Work out the finished part from the listing and answer in its coordinate system (mm). Face numbers are marked on the shaded views. A direction names the side the tool comes from. Coordinates: 2 decimals unless noted, no trailing zeros. Write each loop counter-clockwise with the first axis right and the second up, starting at its lowest first coordinate (ties: lowest second). Pieces come first, ordered by that corner, then holes. Notation, with made-up numbers: (-31.75, 79) - (-23.75, 79) arc R14 cw to (-23.75, 92) - close; hole circle Ø9 at (-38.5, 45.5). An arc over 180 degrees is marked (long way). Use a Markdown table: item, result. Add a question column.
(1) The part is cut by section A-A, the plane y = 14. Give the vertices of the cut face in (x, z), then the cut area to 3 significant figures.
(2) The part is cut by section D-D, the plane y = -5. Give the vertices of the cut face in (x, z).
(3) For a pull along Z with two mould halves and no side action, classify the marked faces 1, 2, 3 and 4 as released by +Z, released by -Z, zero draft, split by the parting line, or undercut.
(4) A tool of negligible diameter and unlimited length cuts with its end or side. For the marked faces 5, 6 and 7, from which of +Z, -Z, +X, -X, +Y, -Y can it reach the whole face along a straight path? Write none if from no direction.
(5) The part is cut by section B-B, the plane z = 5. Give the vertices of the cut face in (x, y).
(6) The part is cut by section C-C, the plane x = 0. Give the vertices of the cut face in (y, z), then the cut area to 3 significant figures.
(7) Find the intervals of material crossed by line 1 (X direction, y = 14, z = 0.5); line 2 (Y direction, x = 3.5, z = -7.25); line 3 (X direction, y = -3, z = -2.25), in increasing order. Write a range as from..to.
(8) Given pin 1 Ø1 at (x, z) = (-3, -2) entering from -Y; pin 2 Ø3 at (x, z) = (-1, 3.5) entering from -Y; pin 3 Ø0.8 at (x, z) = (0, -1) entering from +Y; pin 4 Ø1.6 at (x, z) = (0.5, 1) entering from +Y, each flat-ended and moving along its own axis, determine where each tip first touches the part or whether it passes through.
Autodesk Inventor part; units mm, degrees
ref_plane "YZ Plane" through (0, 0, 0) normal (1, 0, 0) x (0, 1, 0)
ref_plane "XZ Plane" through (0, 0, 0) normal (0, 1, 0) x (-1, 0, 0)
ref_plane "XY Plane" through (0, 0, 0) normal (0, 0, 1) x (1, 0, 0)
sketch "스케치1" plane through (0, 0, 0) normal (0, 1, 0) x (-1, 0, 0)
  arc A0 (5, 6) -> (-5, 6) centre (0, 6) ccw
  arc A1 (-5, -6) -> (5, -6) centre (0, -6) ccw
  line L0 (5, 6) -> (5, -6)
  line L1 (-5, 6) -> (-5, -6)
  point P0 (0, 0)
extrude "돌출1" add sketch "스케치1" along normal blind 20
sketch "스케치2" plane through (0, 20, 0) normal (0, 1, 0) x (1, 0, 0)
  line L0 (0, 0) -> (0, 3)
  line L1 (0, 3) -> (0, -3)
  circle A0 centre (0, 3) radius 1
  circle A1 centre (0, -3) radius 1
  line L2 (1, 3) -> (1, -3)
  line L3 (-1, -3) -> (-1, 3)
  dimension "d10" = 3
  dimension "d11" = 6
  dimension "d12" = 2
  dimension "d13" = 2
extrude "돌출2" cut sketch "스케치2" against normal blind 8
sketch "스케치3" plane through (0, 0, 0) normal (0, -1, 0) x (1, 0, 0)
  line L0 (-3, 0) -> (-3, 5.5316)
  line L1 (-2.6402, 6.2998) -> (-0.6402, 7.9665)
  line L2 (-3, 0) -> (-3, -5.5316)
  line L3 (-2.6402, -6.2998) -> (-0.6402, -7.9665)
  line L4 (3, 0) -> (3, 5.5316)
  line L5 (3, 5.5316) -> (3, -5.5316)
  line L6 (2.6402, -6.2998) -> (0.6402, -7.9665)
  line L7 (2.6402, 6.2998) -> (0.6402, 7.9665)
  arc A0 (-0.6402, -7.9665) -> (0.6402, -7.9665) centre (0, -7.1983) ccw
  arc A1 (2.6402, -6.2998) -> (3, -5.5316) centre (2, -5.5316) ccw
  arc A2 (3, 5.5316) -> (2.6402, 6.2998) centre (2, 5.5316) ccw
  arc A3 (0.6402, 7.9665) -> (-0.6402, 7.9665) centre (0, 7.1983) ccw
  arc A4 (-3, -5.5316) -> (-2.6402, -6.2998) centre (-2, -5.5316) ccw
  arc A5 (-2.6402, 6.2998) -> (-3, 5.5316) centre (-2, 5.5316) ccw
  point P0 (0, 0)
  point P1 (-3, -6)
  point P2 (3, -6)
  dimension "d24" = 1
extrude "돌출3" add sketch "스케치3" along normal blind 8
sketch "스케치4" plane through (0, -8, 0) normal (0, -1, 0) x (1, 0, 0)
  line L0 (0, 0) -> (0, 5)
  line L1 (0, 5) -> (0, -5)
  circle A0 centre (0, 5) radius 1
  circle A1 centre (0, -4.7812) radius 1
  dimension "d27" = 5
  dimension "d28" = 10
  dimension "d29" = 2
  dimension "d30" = 2
extrude "돌출4" add sketch "스케치4" along normal blind 8
ref_plane "작업 평면1" through (0, -16, 4) normal (-1, 0, 0) x (0, 0, 1)
sketch "스케치6" plane through (0, -16, 4) normal (-1, 0, 0) x (0, 0, 1)
  line L0 (0, 0) -> (2, 0)
  line L1 (0, -1) -> (1, -1)
  arc A0 (0, 0) -> (1, -1) centre (1, 0) ccw
  line L2 (1, -1) -> (1, 0)
  line L3 (1, 0) -> (0, 0)
  point P0 (-4, 16)
  point P1 (1, 0)
  point P2 (1, 0)
  dimension "d35" = 1
revolve "회전1" add sketch "스케치6" angle 360 about axis through (0, -17, 5) along (0, 1, 0)
sketch "스케치7" plane through (0, -16, 4) normal (-1, 0, 0) x (0, 0, 1)
  line L0 (-9.7812, 0) -> (-7.7812, 0)
  line L1 (-7.7812, 0) -> (-8.7812, 0)
  line L2 (-8.7812, 0) -> (-8.7812, -1)
  arc A0 (-8.7812, -1) -> (-7.7812, 0) centre (-8.7812, 0) ccw
  point P0 (-4, 16)
  dimension "d37" = 1
  dimension "d38" = 1
revolve "회전2" add sketch "스케치7" angle 360 about axis through (0, -16, -4.7812) along (0, -1, 0)
sketch "스케치8" plane through (0, 12, 0) normal (0, 1, 0) x (1, 0, 0)
  line L0 (0, 0) -> (0, 3)
  line L1 (0, 3) -> (0, -3)
  circle A0 centre (0, -3) radius 0.5
  circle A1 centre (0, 3) radius 0.5
  line L2 (-0.5, -3) -> (-0.5, 3)
  line L3 (0.5, -3) -> (0.5, 3)
  dimension "d40" = 3
  dimension "d41" = 6
  dimension "d42" = 1
  dimension "d43" = 1
extrude "돌출6" add sketch "스케치8" along normal blind 6
properties part number "Ctype addapter"
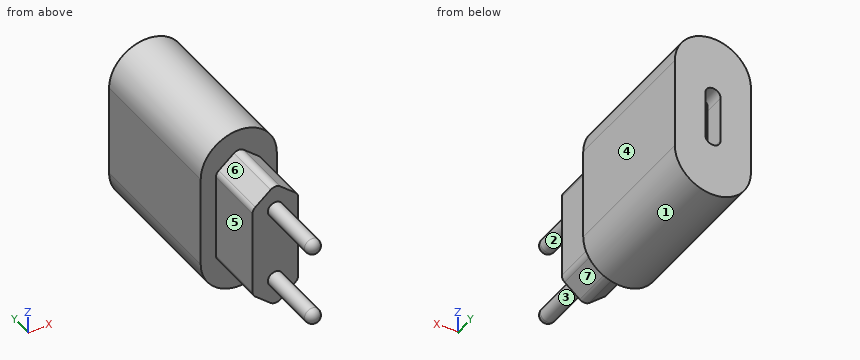
Model answer:
| question | item | result |
|---|---|---|
| 1 | outline | (-5, -6) arc R5 ccw to (5, -6) - (5, 6) arc R5 ccw to (-5, 6) - close; (-0.5, -3) arc R0.5 ccw to (0.5, -3) - (0.5, 3) arc R0.5 ccw to (-0.5, 3) - close; hole (-1, -3) arc R1 ccw to (1, -3) - (1, 3) arc R1 ccw to (-1, 3) - close |
| 1 | area | 190 mm^2 |
| 2 | outline | (-3, -5.53) arc R1 ccw to (-2.64, -6.3) - (-0.64, -7.97) arc R1 ccw to (0.64, -7.97) - (2.64, -6.3) arc R1 ccw to (3, -5.53) - (3, 5.53) arc R1 ccw to (2.64, 6.3) - (0.64, 7.97) arc R1 ccw to (-0.64, 7.97) - (-2.64, 6.3) arc R1 ccw to (-3, 5.53) - close |
| 3 | face 1 | released by -Z |
| 3 | face 2 | undercut |
| 3 | face 3 | undercut |
| 3 | face 4 | zero draft |
| 4 | face 5 | +Z, -Z, -X, -Y |
| 4 | face 6 | +Z, -X, -Y |
| 4 | face 7 | -Z, +X, -Y |
| 5 | outline | (-5, 0) - (-3, 0) - (-3, -8) - (-1, -8) - (-1, -16) arc R1 ccw to (1, -16) - (1, -8) - (3, -8) - (3, 0) - (5, 0) - (5, 20) - (-5, 20) - close |
| 6 | outline | (-16, -5.78) - (-8, -5.78) - (-8, -8.2) - (0, -8.2) - (0, -11) - (20, -11) - (20, -4) - (12, -4) - (12, -3.5) - (18, -3.5) - (18, 3.5) - (12, 3.5) - (12, 4) - (20, 4) - (20, 11) - (0, 11) - (0, 8.2) - (-8, 8.2) - (-8, 6) - (-16, 6) arc R1 ccw to (-16, 4) - (-8, 4) - (-8, -3.78) - (-16, -3.78) arc R1 ccw to start |
| 6 | area | 584 mm^2 |
| 7 | line 1 | -5..-1, -0.5..0.5, 1..5 |
| 7 | line 2 | 0..20 |
| 7 | line 3 | -3..3 |
| 8 | pin 1 | y = -8 |
| 8 | pin 2 | y = -16.95 |
| 8 | pin 3 | y = 18 |
| 8 | pin 4 | y = 20 |
